Here's how the part is built. I have some questions about the finished solid (model axes, mm). Give positions to 0.01 mm unless a question says otherwise; leave off trailing zeros. Return JSON: item names as keys, results as strings. Group by question number.
(1) If we section it at A-A (z = 0): State how many separate pieces and enclosed holes the cut face has, then the cut area to 3 significant figures.
(2) For P1, Ø1.1, axis at x = 13.5, z = 1, coming from the +Y side; P2, Ø1, axis at x = -62, z = -1, coming from the +Y side; P3, Ø2, axis at y = 7.5, z = -5, coming from the -X side, each with a flat end and sliding along its axis, tell me the tip position at first contact or that it passes through.
(3) I need wall thicknesses on probe 1 along X at (y, z) = (-2.35, 0); probe 2 along Z at (x, y) = (82, -2.9); probe 3 along X at (y, z) = (9.5, -2.5). Which ranges of each line are inside material? Lowest first, please. Write a range as [from, to].
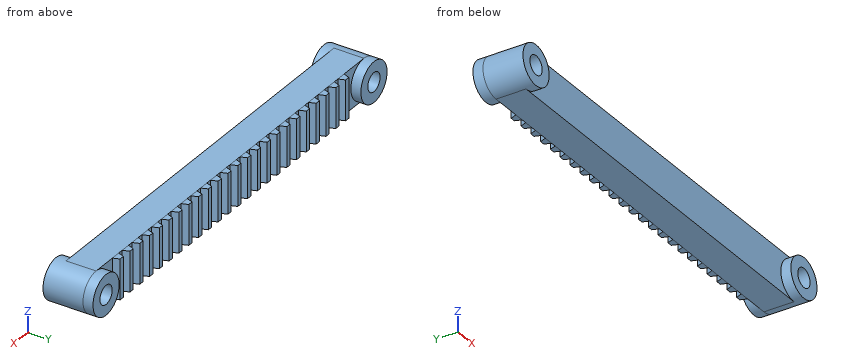
```python
from build123d import *

# Parameters (mm, degrees)
SKETCH1_W                = 164
SKETCH1_H                = 16
BOSS_EXTRUDE1_DEPTH      = 12
SKETCH2_R                = 8
BOSS_EXTRUDE2_DEPTH      = 4
BOSS_EXTRUDE2_DEPTH_BACK = 16
BOSS_EXTRUDE3_DEPTH      = 16
LPATTERN1_COUNT          = 24
LPATTERN1_PITCH          = 6
SKETCH4_R                = 3.75
CUT_EXTRUDE1_DEPTH       = 5
CUT_EXTRUDE1_DEPTH_BACK  = 17


with BuildPart() as part:
    # Sketch1 → Boss-Extrude1 (new body)
    with BuildSketch(Plane(origin=(0, 0, 0), x_dir=(1, 0, 0), z_dir=(0, 1, 0))):
        Rectangle(SKETCH1_W, SKETCH1_H)
    extrude(amount=BOSS_EXTRUDE1_DEPTH)

    # Sketch2 → Boss-Extrude2 (add, two sides)
    with BuildSketch(Plane(origin=(0, 12, 0), x_dir=(1, 0, 0), z_dir=(0, 1, 0))) as boss_extrude2_sk:
        with Locations((-82, 0)):
            Circle(SKETCH2_R)
        with Locations((82, 0)):
            Circle(SKETCH2_R)
    extrude(amount=BOSS_EXTRUDE2_DEPTH)
    extrude(boss_extrude2_sk.sketch, amount=-BOSS_EXTRUDE2_DEPTH_BACK)

    # Sketch3 → Boss-Extrude3 (add)
    with BuildSketch(Plane.XY.offset(8)):
        Polygon((68.180148829, 12), (72, 12), (71.090074414, 14.5), (69.090074414, 14.5), align=None)
    boss_extrude3 = extrude(amount=-BOSS_EXTRUDE3_DEPTH)

    # LPattern1: Boss-Extrude3 ×24
    with Locations(*[(-i * LPATTERN1_PITCH, 0, 0) for i in range(1, LPATTERN1_COUNT)]):
        add(boss_extrude3)

    # Sketch4 → Cut-Extrude1 (cut, two sides)
    with BuildSketch(Plane.XZ) as cut_extrude1_sk:
        with Locations((-82, 0)):
            Circle(SKETCH4_R)
        with Locations((82, 0)):
            Circle(SKETCH4_R)
    extrude(amount=CUT_EXTRUDE1_DEPTH, mode=Mode.SUBTRACT)
    extrude(cut_extrude1_sk.sketch, amount=-CUT_EXTRUDE1_DEPTH_BACK, mode=Mode.SUBTRACT)


solid = part.part
```
Values:
{
 "1": {"separate pieces": "3", "enclosed holes": "0", "area": "2,290 mm2"},
 "2": {"P1": "y = 12", "P2": "y = 14.5", "P3": "x = -88.93"},
 "3": {"probe 1": "[-90, -85.75], [-78.25, -74], [74, 78.25], [85.75, 90]", "probe 2": "[-8, -3.75], [3.75, 8]", "probe 3": "[-89.6, -84.8], [-79.2, 79.2], [84.8, 89.6]"}
}
